from build123d import *

# Parameters (mm, degrees)
EXTRUDE_1_DEPTH     = 15
SKETCH_2_R          = 25
EXTRUDE_2_DEPTH     = 10
CUT_EXTRUDE_1_DEPTH = 121
SKETCH_4_R          = 7
CUT_EXTRUDE_2_DEPTH = 121


with BuildPart() as part:
    # 草图1 → 凸台-拉伸1 (new body)
    with BuildSketch(Plane.XY):
        Polygon((50, 0), (60, 0), (48.29629, 12.94095), (57.95555, 15.52914), (43.30127, 25), (51.96152, 30), (35.35534, 35.35534), (42.42641, 42.42641), (25, 43.30127), (30, 51.96152), (12.94095, 48.29629), (15.52914, 57.95555), (0, 50), (0, 60), (-12.94095, 48.29629), (-15.52914, 57.95555), (-25, 43.30127), (-30, 51.96152), (-35.35534, 35.35534), (-42.42641, 42.42641), (-43.30127, 25), (-51.96152, 30), (-48.29629, 12.94095), (-57.95555, 15.52914), (-50, 0), (-60, 0), (-48.29629, -12.94095), (-57.95555, -15.52914), (-43.30127, -25), (-51.96152, -30), (-35.35534, -35.35534), (-42.42641, -42.42641), (-25, -43.30127), (-30, -51.96152), (-12.94095, -48.29629), (-15.52914, -57.95555), (0, -50), (0, -60), (12.94095, -48.29629), (15.52914, -57.95555), (25, -43.30127), (30, -51.96152), (35.35534, -35.35534), (42.42641, -42.42641), (43.30127, -25), (51.96152, -30), (48.29629, -12.94095), (57.95555, -15.52914), align=None)
    extrude(amount=EXTRUDE_1_DEPTH)

    # 草图2 → 凸台-拉伸2 (add)
    with BuildSketch(Plane.XY.offset(15)):
        Circle(SKETCH_2_R)
    extrude(amount=EXTRUDE_2_DEPTH)

    # 草图3 → 切除-拉伸1 (cut, symmetric)
    with BuildSketch(Plane.XY.offset(25)):
        Polygon((12, 6.92820323), (0, 13.856406461), (-12, 6.92820323), (-12, -6.92820323), (0, -13.856406461), (12, -6.92820323), align=None)
    extrude(amount=CUT_EXTRUDE_1_DEPTH, both=True, mode=Mode.SUBTRACT)

    # 草图4 → 切除-拉伸2 (cut, symmetric)
    with BuildSketch(Plane.XY.offset(15)):
        with Locations((33, 0)):
            Circle(SKETCH_4_R)
        with Locations((16.5, 28.578838)):
            Circle(SKETCH_4_R)
        with Locations((-16.5, 28.578838)):
            Circle(SKETCH_4_R)
        with Locations((-33, 0)):
            Circle(SKETCH_4_R)
        with Locations((-16.5, -28.578838)):
            Circle(SKETCH_4_R)
        with Locations((16.5, -28.578838)):
            Circle(SKETCH_4_R)
    extrude(amount=CUT_EXTRUDE_2_DEPTH, both=True, mode=Mode.SUBTRACT)


solid = part.part
Work out the finished part from the listing and answer in its coordinate system (mm). A direction names the side the tool comes from. Coordinates: 2 decimals unless noted, no trailing zeros. Write each loop counter-clockwise with the first axis right and the second up, starting at its lowest first coordinate (ties: lowest second). Pieces come first, ordered by that corner, then holes.
1. The part is cut by section B-B, the plane x = -32.5. Write down the section's boundary in (y, z), and give its area (3 significant figures).
Results list:
outline: (-42.92, 0) - (-6.98, 0) - (-6.98, 15) - (-42.92, 15) - close; (6.98, 0) - (44.21, 0) - (44.21, 15) - (6.98, 15) - close
area: 1,100 mm2
2. For a pull along X with two mould halves and no side action, classify faces 6 (the flat face through (47.571, 27.465, 7.395)), 7 (the flat face through (27.465, -47.571, 7.395)), 8 (the flat face through (-54.23, -6.38, 7.4)) as +X half, -X half, draft (parallel to the pull), parting line (faces both ways), or undercut.
Results list:
face 6: +X half
face 7: undercut
face 8: -X half
3. For faces 1 (the flat face through (6.084, 10.344, 12.675)), 2 (the flat face through (42.858, -33.835, 7.395)), 3 (the flat face through (-50.73, -20.2, 7.4)), 4 (the flat face through (-20.2, 50.73, 7.4)), 5 (the flat face through (43.77, 32.64, 7.4)), determine the directions among +Z, -Z, +X, -X, +Y, -Y from which every point of the face is accessible in a straight line to the end or side of a thin tool.
Results list:
face 1: +Z, -Z
face 2: +Z, -Z, -Y
face 3: +Z, -Z, -X
face 4: +Z, -Z, +Y
face 5: +Z, -Z, +X
4. Flat-ended cylindrical pins translate along their axes: pin 1 (5 mm diameter, centred on x = 31, y = -42, fed in from +Z); pin 2 (1.5 mm diameter, centred on y = 11, z = 14, fed in from +X); pin 3 (11 mm diameter, centred on x = 16.5, y = 28.58, fed in from +Z) (1 decimal); pin 4 (3 mm diameter, centred on x = -54, z = 8.5, fed in from +Y). Find the tip coordinate at first contact, or state that the pin passes through.
Results list:
pin 1: stops at z = 15
pin 2: stops at x = 50.73
pin 3: passes through
pin 4: stops at y = 14.87
5. Consider line 1 along Y through (x, z) = (16.5, 10.5); line 2 along Y through (x, z) = (-16.5, 11.25); line 3 along X through (y, z) = (25.5, 14). Determine where each line is inside the solid, lowest interval first.
Results list:
line 1: y = -56.45 to -35.58, -21.58 to 21.58, 35.58 to 49.06
line 2: y = -49.06 to -35.58, -21.58 to 21.58, 35.58 to 56.45
line 3: x = -50.99 to -44.17, -43.28 to -22.79, -10.21 to 10.21, 22.79 to 44.17
6. The part is cut by section A-A, the plane z = 23. Write down the section's boundary in (x, y).
Results list:
outline: circle Ø50 at (0, 0); hole (-12, -6.93) - (0, -13.86) - (12, -6.93) - (12, 6.93) - (0, 13.86) - (-12, 6.93) - close
7. The part is cut by section D-D, the plane x = 5. Write down the section's boundary in (y, z), and give its area (3 significant figures).
Results list:
outline: (-55.48, 0) - (-10.97, 0) - (-10.97, 25) - (-24.49, 25) - (-24.49, 15) - (-55.48, 15) - close; (10.97, 0) - (52.56, 0) - (52.56, 15) - (24.49, 15) - (24.49, 25) - (10.97, 25) - close
area: 1,560 mm2
8. The part is cut by section C-C, the plane z = 7.75. State how many separate pieces and enclosed holes the cut face has, and give its area (3 significant figures).
Results list:
separate pieces: 1
enclosed holes: 7
area: 7,900 mm2
